from build123d import *

# Parameters (mm, degrees)
SKETCH1_W           = 100
SKETCH1_H           = 82
BOSS_EXTRUDE1_DEPTH = 2
CHAMFER1_SIZE       = 4
SKETCH2_R           = 1.6
CUT_EXTRUDE1_DEPTH  = 130.336769714
SKETCH3_W           = 100
SKETCH3_H           = 2
BOSS_EXTRUDE2_DEPTH = 30
SKETCH4_W           = 20
SKETCH4_H           = 2
CUT_EXTRUDE2_DEPTH  = 130.336769714
BOSS_EXTRUDE3_DEPTH = 4
SKETCH6_R           = 1.4
CUT_EXTRUDE3_DEPTH  = 130.460418661
SKETCH7_W           = 20
SKETCH7_H           = 10
CUT_EXTRUDE4_DEPTH  = 130.383151917


with BuildPart() as part:
    # Sketch1 → Boss-Extrude1 (new body)
    with BuildSketch(Plane(origin=(0, 0, 0), x_dir=(1, 0, 0), z_dir=(0, 1, 0))):
        with Locations((50, 41)):
            Rectangle(SKETCH1_W, SKETCH1_H)
    extrude(amount=BOSS_EXTRUDE1_DEPTH)

    # Chamfer1
    chamfer1_edges = [part.edges().sort_by_distance(p)[0] for p in [
        (0, 1, -82),
        (100, 1, -82),
    ]]
    chamfer(chamfer1_edges, length=CHAMFER1_SIZE)

    # Sketch2 → Cut-Extrude1 (cut, through all)
    with BuildSketch(Plane(origin=(0, 2, 0), x_dir=(1, 0, 0), z_dir=(0, 1, 0))):
        with Locations(Location((8, 78, 0), (0, 0, 270))):
            Circle(SKETCH2_R)
        with Locations(Location((92, 78, 0), (0, 0, 270))):
            Circle(SKETCH2_R)
        with Locations(Location((97, 4, 0), (0, 0, 270))):
            Circle(SKETCH2_R)
        with Locations(Location((3, 4, 0), (0, 0, 270))):
            Circle(SKETCH2_R)
    extrude(amount=-CUT_EXTRUDE1_DEPTH, mode=Mode.SUBTRACT)

    # Sketch3 → Boss-Extrude2 (add)
    with BuildSketch(Plane.XY):
        with Locations((50, 1)):
            Rectangle(SKETCH3_W, SKETCH3_H)
    extrude(amount=BOSS_EXTRUDE2_DEPTH)

    # Sketch4 → Cut-Extrude2 (cut, through all)
    with BuildSketch(Plane(origin=(0, 2, 0), x_dir=(1, 0, 0), z_dir=(0, 1, 0))):
        with Locations((25, -27)):
            Rectangle(SKETCH4_W, SKETCH4_H)
        with Locations((75, -27)):
            Rectangle(SKETCH4_W, SKETCH4_H)
        with Locations((25, 10)):
            Rectangle(SKETCH4_W, SKETCH4_H)
        with Locations((75, 10)):
            Rectangle(SKETCH4_W, SKETCH4_H)
    extrude(amount=-CUT_EXTRUDE2_DEPTH, mode=Mode.SUBTRACT)

    # Sketch5 → Boss-Extrude3 (add)
    with BuildSketch(Plane(origin=(0, 2, 0), x_dir=(1, 0, 0), z_dir=(0, 1, 0))):
        Polygon((10, 68.035898385), (13, 69.767949192), (13, 73.232050808), (10, 74.964101615), (7, 73.232050808), (7, 69.767949192), align=None)
        Polygon((10, 25.964101615), (7, 24.232050808), (7, 20.767949192), (10, 19.035898385), (13, 20.767949192), (13, 24.232050808), align=None)
        Polygon((68, 25.964101615), (65, 24.232050808), (65, 20.767949192), (68, 19.035898385), (71, 20.767949192), (71, 24.232050808), align=None)
        Polygon((68, 68.035898385), (71, 69.767949192), (71, 73.232050808), (68, 74.964101615), (65, 73.232050808), (65, 69.767949192), align=None)
    extrude(amount=BOSS_EXTRUDE3_DEPTH)

    # Sketch6 → Cut-Extrude3 (cut, through all)
    with BuildSketch(Plane(origin=(0, 6, 0), x_dir=(1, 0, 0), z_dir=(0, 1, 0))):
        with Locations(Location((10, 71.5, 0), (0, 0, 270))):
            Circle(SKETCH6_R)
        with Locations(Location((68, 71.5, 0), (0, 0, 270))):
            Circle(SKETCH6_R)
        with Locations(Location((68, 22.5, 0), (0, 0, 270))):
            Circle(SKETCH6_R)
        with Locations(Location((10, 22.5, 0), (0, 0, 270))):
            Circle(SKETCH6_R)
    extrude(amount=-CUT_EXTRUDE3_DEPTH, mode=Mode.SUBTRACT)

    # Sketch7 → Cut-Extrude4 (cut, through all)
    with BuildSketch(Plane(origin=(0, 2, 0), x_dir=(1, 0, 0), z_dir=(0, 1, 0))):
        with Locations((50, 14)):
            Rectangle(SKETCH7_W, SKETCH7_H)
    extrude(amount=-CUT_EXTRUDE4_DEPTH, mode=Mode.SUBTRACT)


solid = part.part
Part model, mm, in its own coordinate system. A direction names the side the tool comes from. Give positions to 0.01 mm unless a question says otherwise; leave off trailing zeros. Loops run counter-clockwise (first coordinate to the right, second up) from the corner with the lowest first, then second, coordinate; pieces in that order, holes last. Notation, with made-up numbers: M 51.5,74 L 66.5,74 A27 cw 66.5,96 Z; hole C -21,-1.75 d9. An arc over 180 degrees is marked long. Put each result on its own line as item: value. Start each with the question number.
1) Probe probe 1 along Z at (x, y) = (27, 1.05); probe 2 along X at (y, z) = (1.3, -78); probe 3 along X at (y, z) = (1.8, -22.5). List the from-to ranges inside material, lowest first.
2) 3-axis set-ups, long thin cutter, end or side, ignore diameter. For faces 5 (the flat face through (69.5, 4, -68.9)), 6 (the flat face through (65, 4, -72)), 7 (the flat face through (71, 4, -22)): which of +Z, -Z, +X, -X, +Y, -Y reach the whole face in a straight line?
3) Saw through at C-C (z = -71.5). List the corners of the cut face in (x, y).
4) Saw through at D-D (x = 45.5). List the corners of the cut face in (y, z).
5) Saw through at B-B (x = 28.5). List the corners of the cut face in (y, z).
6) Pull direction X, two halves, no side cores. Call faces 1 (the flat face through (69.5, 4, -74.1)), 2 (the flat face through (66.5, 4, -74.1)), 3 (the flat face through (2, 1, -80)), 4 (the flat face through (49, 0, -27)): +X half, -X half, draft (parallel to the pull), parting line (faces both ways), or undercut.
7) Flat gauge pins, fed straight in: pin 1 (4 mm diameter, centred on x = 53, z = -65.5, fed in from +Y); pin 2 (1 mm diameter, centred on y = 4.5, z = -22.5, fed in from -X). Where does each tip first touch, or does it go through?
8) Saw through at A-A (y = 3.45). List the corners of the cut face in (x, z), then the cut area to 3 significant figures.
Numbers:
1. probe 1: -82 to -11, -9 to 26, 28 to 30
1. probe 2: 0 to 6.4, 9.6 to 90.4, 93.6 to 100
1. probe 3: 0 to 8.6, 11.4 to 66.6, 69.4 to 100
2. face 5: +X, +Y
2. face 6: +Z, -Z, +Y
2. face 7: +Z, -Z, +X, +Y
3. outline: M 0,0 L 8.6,0 L 8.6,6 L 7,6 L 7,2 L 0,2 Z; M 11.4,0 L 66.6,0 L 66.6,6 L 65,6 L 65,2 L 13,2 L 13,6 L 11.4,6 Z; M 69.4,0 L 100,0 L 100,2 L 71,2 L 71,6 L 69.4,6 Z
4. outline: M 0,-82 L 2,-82 L 2,-19 L 0,-19 Z; M 0,-9 L 2,-9 L 2,30 L 0,30 Z
5. outline: M 0,-82 L 2,-82 L 2,-11 L 0,-11 Z; M 0,-9 L 2,-9 L 2,26 L 0,26 Z; M 0,28 L 2,28 L 2,30 L 0,30 Z
6. face 1: +X half
6. face 2: undercut
6. face 3: -X half
6. face 4: draft
7. pin 1: y = 2
7. pin 2: x = 7
8. outline: M 7,-73.23 L 10,-74.96 L 13,-73.23 L 13,-69.77 L 10,-68.04 L 7,-69.77 Z; M 7,-24.23 L 10,-25.96 L 13,-24.23 L 13,-20.77 L 10,-19.04 L 7,-20.77 Z; M 65,-73.23 L 68,-74.96 L 71,-73.23 L 71,-69.77 L 68,-68.04 L 65,-69.77 Z; M 65,-24.23 L 68,-25.96 L 71,-24.23 L 71,-20.77 L 68,-19.04 L 65,-20.77 Z; hole C 10,-71.5 d2.8; hole C 10,-22.5 d2.8; hole C 68,-71.5 d2.8; hole C 68,-22.5 d2.8
8. area: 100 mm^2
